```python
from build123d import *

# Parameters (mm, degrees)
BOSS_EXTRUDE1_DEPTH      = 50
SKETCH2_R                = 3.25
CUT_EXTRUDE1_DEPTH       = 103.805641869
CHAMFER1_SIZE            = 2
SKETCH3_R                = 4.5
CUT_EXTRUDE2_DEPTH       = 86.469292731
CUT_EXTRUDE3_DEPTH       = 2.5
CHAMFER2_SIZE            = 0.5
BOSS_EXTRUDE2_DEPTH      = 5
CHAMFER2_OF_MIRROR1_SIZE = 0.5
CUT_EXTRUDE4_DEPTH       = 4
CHAMFER3_SIZE            = 0.3


# Read off the part's stored shape, not the designer's step: Mirror2
with BuildPart() as part:
    # Sketch1 → Boss-Extrude1 (new, symmetric)
    with BuildSketch(Plane.XY):
        with BuildLine():
            Line((-25, 0), (25, 0))
            ThreePointArc((25, 0), (29.242640687, 1.757359313), (31, 6))
            Line((31, 6), (31, 65))
            Line((31, 65), (28, 65))
            Line((28, 65), (28, 6))
            ThreePointArc((28, 6), (27.121320344, 3.878679656), (25, 3))
            Line((25, 3), (-25, 3))
            ThreePointArc((-25, 3), (-27.121320344, 3.878679656), (-28, 6))
            Line((-28, 6), (-28, 65))
            Line((-28, 65), (-31, 65))
            Line((-31, 65), (-31, 6))
            ThreePointArc((-31, 6), (-29.242640687, 1.757359313), (-25, 0))
        make_face()
    extrude(amount=BOSS_EXTRUDE1_DEPTH, both=True)

    # Sketch2 → Cut-Extrude1 (cut, through all)
    with BuildSketch(Plane(origin=(31, 0, 0), x_dir=(0, 0, -1), z_dir=(1, 0, 0))):
        with Locations((-37.5, 58)):
            Circle(SKETCH2_R)
        with Locations((37.5, 58)):
            Circle(SKETCH2_R)
    extrude(amount=-CUT_EXTRUDE1_DEPTH, mode=Mode.SUBTRACT)

    # Chamfer1
    chamfer1_edges = [part.edges().sort_by_distance(p)[0] for p in [
        (-29.5, 65, -50),
        (29.5, 65, -50),
        (29.5, 65, 50),
        (-29.5, 65, 50),
    ]]
    chamfer(chamfer1_edges, length=CHAMFER1_SIZE)

    # Sketch3 → Cut-Extrude2 (cut, through all)
    with BuildSketch(Plane(origin=(0, 3, 0), x_dir=(1, 0, 0), z_dir=(0, 1, 0))):
        with Locations(Location((-15, 0, 0), (0, 0, 180))):
            Circle(SKETCH3_R)
        with Locations(Location((15, 0, 0), (0, 0, 180))):
            Circle(SKETCH3_R)
    extrude(amount=-CUT_EXTRUDE2_DEPTH, mode=Mode.SUBTRACT)

    # Sketch4 → Revolve1 (revolve)
    with BuildSketch(Plane(origin=(0, 58, 0), x_dir=(1, 0, 0), z_dir=(0, 1, 0)), mode=Mode.PRIVATE) as revolve1_sk:
        Polygon((23, -40), (31, -40), (31, -41.75), (36, -41.75), (36, -37.5), (23, -37.5), align=None)
    revolve1 = revolve(revolve1_sk.sketch.rotate(Axis((36, 58, 37.5), (-1, 0, 0)), 180), axis=Axis((36, 58, 37.5), (-1, 0, 0)))

    # Sketch5 → Cut-Extrude3 (cut)
    with BuildSketch(Plane(origin=(36, 0, 0), x_dir=(0, 0, -1), z_dir=(1, 0, 0))):
        Polygon((-37.5, 60.309401077), (-39.5, 59.154700538), (-39.5, 56.845299462), (-37.5, 55.690598923), (-35.5, 56.845299462), (-35.5, 59.154700538), align=None)
    cut_extrude3 = extrude(amount=-CUT_EXTRUDE3_DEPTH, mode=Mode.SUBTRACT)

    # Chamfer2
    chamfer2_edges = [part.edges().sort_by_distance(p)[0] for p in [
        (36, 58, 41.75),
    ]]
    chamfer(chamfer2_edges, length=CHAMFER2_SIZE)

    # Sketch6 → Boss-Extrude2 (add, symmetric)
    with BuildSketch(Plane.XY.offset(37.5)):
        with BuildLine():
            Line((22.2, 60.743829885), (22.2, 55.256170115))
            ThreePointArc((22.2, 55.256170115), (22.23389675, 55.117645531), (22.327927069, 55.010424502))
            Line((22.327927069, 55.010424502), (25.140026938, 53.041370976))
            ThreePointArc((25.140026938, 53.041370976), (25.376869026, 53.025847525), (25.5, 53.228761091))
            Line((25.5, 53.228761091), (25.5, 55.1))
            Line((25.5, 55.1), (26.1, 55.1))
            ThreePointArc((26.1, 55.1), (26.241421356, 55.158578644), (26.3, 55.3))
            Line((26.3, 55.3), (26.3, 60.7))
            ThreePointArc((26.3, 60.7), (26.241421356, 60.841421356), (26.1, 60.9))
            Line((26.1, 60.9), (25.5, 60.9))
            Line((25.5, 60.9), (25.5, 62.771238909))
            ThreePointArc((25.5, 62.771238909), (25.376869026, 62.974152475), (25.140026938, 62.958629024))
            Line((25.140026938, 62.958629024), (22.327927069, 60.989575498))
            ThreePointArc((22.327927069, 60.989575498), (22.23389675, 60.882354469), (22.2, 60.743829885))
        make_face()
    boss_extrude2 = extrude(amount=BOSS_EXTRUDE2_DEPTH, both=True)

    # Mirror1: Revolve1, Cut-Extrude3, Boss-Extrude2 across plane
    add(revolve1.mirror(Plane.XY))
    add(cut_extrude3.mirror(Plane.XY), mode=Mode.SUBTRACT)
    add(boss_extrude2.mirror(Plane.XY))

    # Chamfer2 of Mirror1
    chamfer2_of_mirror1_edges = [part.edges().sort_by_distance(p)[0] for p in [
        (36, 58, -41.75),
    ]]
    chamfer(chamfer2_of_mirror1_edges, length=CHAMFER2_OF_MIRROR1_SIZE)

    # Sketch7 → Revolve2 (revolve)
    with BuildSketch(Plane.XY, mode=Mode.PRIVATE) as revolve2_sk:
        Polygon((18, 11), (21.5, 11), (21.5, 3), (19, 3), (19, -22), (15, -22), (15, 5.267949192), (18, 7), align=None)
    revolve(revolve2_sk.sketch.rotate(Axis((15, 11, 0), (0, -1, 0)), 180), axis=Axis((15, 11, 0), (0, -1, 0)))

    # Sketch8 → Cut-Extrude4 (cut)
    with BuildSketch(Plane(origin=(0, 11, 0), x_dir=(1, 0, 0), z_dir=(0, 1, 0))):
        Polygon((15, 3.464101615), (12, 1.732050808), (12, -1.732050808), (15, -3.464101615), (18, -1.732050808), (18, 1.732050808), align=None)
    extrude(amount=-CUT_EXTRUDE4_DEPTH, mode=Mode.SUBTRACT)

    # Chamfer3
    chamfer3_edges = [part.edges().sort_by_distance(p)[0] for p in [
        (21.5, 11, 0),
    ]]
    chamfer(chamfer3_edges, length=CHAMFER3_SIZE)

    # Mirror2: part across plane


with BuildPart() as part_1:
    add(part.part)
    add(part.part.mirror(Plane(origin=(0, 0, 0), x_dir=(0, 0, 1), z_dir=(1, 0, 0))))


solid = part_1.part
```
Work out the finished part from the listing and answer in its coordinate system (mm). A direction names the side the tool comes from. Coordinates: 2 decimals unless noted, no trailing zeros. Write each loop counter-clockwise with the first axis right and the second up, starting at its lowest first coordinate (ties: lowest second). Pieces come first, ordered by that corner, then holes.
Q1. A cutting plane is placed at B-B, the plane z = -8. Give the vertices of the cut face in (x, y), then the cut area to 3 significant figures.
Q2. A cutting plane is placed at D-D, the plane y = -12. Give the vertices of the cut face in (x, z), then the cut area to 3 significant figures.
Q3. Find the intervals of material crossed by line 1 (X direction, y = 44.5, z = 15.5); line 2 (Y direction, x = -29.3, z = -37.5); line 3 (Y direction, x = -29.6, z = 37.5), in increasing order.
Q4. A cutting plane is placed at C-C, the plane x = -1. Give the vertices of the cut face in (y, z), then the cut area to 3 significant figures.
Q5. Determine the mould class of faces 6 (the face through (19.496, 1.521, 0.198)), 7 (the face through (35, 58, 35.5)), 8 (the face through (31, 35, 1)) for opening direction X: released by +X, released by -X, zero draft, split by the parting line, or undercut.
Q6. Which of the six approach directions +Z, -Z, +X, -X, +Y, -Y give full straight-line access (tool end or side, diameter ignored) to faces 1 (the face through (35, 58, 39.5)), 2 (the face through (24, 58, -42.5)), 3 (the face through (-28.683, 57.249, -35.115)), 4 (the face through (18, 9, 0)), 5 (the face through (22.2, 58, -38))?
Q7. Each of these flat-tipped pins is pushed along its axis until it touches: pin 1 Ø17.5 at (y, z) = (50, -15.5) entering from +X; pin 2 Ø4 at (y, z) = (1, -10) entering from +X; pin 3 Ø3 at (x, z) = (19, 12) entering from +Y. Where does it stop, or does it pass through?
Q8. A cutting plane is placed at A-A, the plane y = 19.5. Give the vertices of the cut face in (x, z).
Findings below:
1. outline: (-31, 6) arc R6 ccw to (-25, 0) - (25, 0) arc R6 ccw to (31, 6) - (31, 65) - (28, 65) - (28, 6) arc R3 cw to (25, 3) - (-25, 3) arc R3 cw to (-28, 6) - (-28, 65) - (-31, 65) - close
1. area: 546 mm2
2. outline: circle Ø8 at (-15, 0); circle Ø8 at (15, 0)
2. area: 101 mm2
3. line 1: x = -31 to -28, 28 to 31
3. line 2: y = 1.82 to 54.75, 55.5 to 60.5, 61.25 to 65
3. line 3: y = 2.15 to 54.75, 55.5 to 60.5, 61.25 to 65
4. outline: (0, -50) - (3, -50) - (3, 50) - (0, 50) - close
4. area: 300 mm2
5. face 6: undercut
5. face 7: zero draft
5. face 8: released by +X
6. face 1: +X
6. face 2: -Z, +Y
6. face 3: none
6. face 4: +Y
6. face 5: +Z, -Z, +Y
7. pin 1: stops at x = 31
7. pin 2: stops at x = 30.2
7. pin 3: stops at y = 3
8. outline: (-31, -50) - (-28, -50) - (-28, 50) - (-31, 50) - close; (28, -50) - (31, -50) - (31, 50) - (28, 50) - close
